Autodesk Inventor part; units mm, degrees
ref_plane "YZ Plane" through (0, 0, 0) normal (1, 0, 0) x (0, 1, 0)
ref_plane "XZ Plane" through (0, 0, 0) normal (0, 1, 0) x (-1, 0, 0)
ref_plane "XY Plane" through (0, 0, 0) normal (0, 0, 1) x (1, 0, 0)
sketch "Sketch1" plane through (0, 0, 0) normal (0, 1, 0) x (-1, 0, 0)
  line L0 (0, 0) -> (0, 15.8369)
  line L1 (0, 0) -> (20.1574, 0)
  line L2 (20.1574, 0) -> (20.1574, 7.7978)
  line L3 (20.1574, 7.7978) -> (0, 15.8369)
  dimension "d0" = 15.8369
  dimension "d1" = 20.1574
  dimension "d2" = 7.7978
extrude "Extrusion1" add sketch "Sketch1" along normal blind 3.236
sketch "Sketch2" plane through (0, 3.236, 0) normal (0, 1, 0) x (1, 0, 0)
  line L0 (-20.1574, -7.7978) -> (0, -15.8369)
  line L1 (-20.1574, 0) -> (-20.1574, -7.7978)
  line L2 (0, 0) -> (-20.1574, 0)
  line L3 (-20.1574, 0) -> (-20.1574, -7.7978)
  circle A0 centre (-16.2585, -3.8989) radius 2.4498
  dimension "d7" = 4.8997
extrude "Extrusion2" add sketch "Sketch2" along normal blind 1.9837
pattern_linear "Rectangular Pattern1" count 3 spacing 6.223 along (1, 0, 0) of "Extrusion2"
properties part number "other diagonal piece"
Verification items for the finished model (mm, model axes). A direction names the side the tool comes from. Coordinates: 2 decimals unless noted, no trailing zeros. Loops run counter-clockwise (first coordinate to the right, second up) from the corner with the lowest first, then second, coordinate; pieces in that order, holes last. Notation, with made-up numbers: (-33, 42.5) -> (-4, 42.5) arc R28 ccw to (-4, 70.5) -> close; hole circle Ø2 at (-32, -27.75). An arc over 180 degrees is marked (long way). Answer in a Markdown table with one row per item.
1) Scan lines: line 1 along X through (y, z) = (4.65, 4); line 2 along Y through (x, z) = (-7.5, 11); line 3 along Z through (x, y) = (-10.75, 4.85). Record each from-to range of solid material in increasing order. Write a range as from..to.
The answers:
| item | result |
|---|---|
| line 1 | x = -18.71..-13.81, -12.48..-7.59, -6.26..-1.36 |
| line 2 | y = 0..3.24 |
| line 3 | z = 1.56..6.24 |
2) Section check B-B (y = 3.85). Record the cut outline in (x, z).
The answers:
| item | result |
|---|---|
| outline | circle Ø4.9 at (-16.26, 3.9); circle Ø4.9 at (-10.04, 3.9); circle Ø4.9 at (-3.81, 3.9) |
3) Section check A-A (x = -2.75). Record the cut outline in (y, z).
The answers:
| item | result |
|---|---|
| outline | (0, 0) -> (3.24, 0) -> (3.24, 1.69) -> (5.22, 1.69) -> (5.22, 6.11) -> (3.24, 6.11) -> (3.24, 14.74) -> (0, 14.74) -> close |
4) Draft check along X on faces 1 (the face through (-10, 2, 0)), 2 (the face through (-4.13, 4.21, 6.33)), 3 (the face through (0, 2, 8)), 4 (the face through (-20.157, 2, 4)). Enter one of: released by +X, released by -X, zero draft, split by the parting line, or undercut.
The answers:
| item | result |
|---|---|
| face 1 | zero draft |
| face 2 | undercut |
| face 3 | released by +X |
| face 4 | released by -X |
5) Access from +Z, -Z, +X, -X, +Y, -Y to the whole of each face (thin tool, end or side, straight path). Record for faces 5 (the face through (-18.064, 4.214, 5.555)), 6 (the face through (-4, 5.22, 4)).
The answers:
| item | result |
|---|---|
| face 5 | +Y |
| face 6 | +Z, -Z, +X, -X, +Y |
6) Section check D-D (y = 1.35). Record the cut outline in (x, z).
The answers:
| item | result |
|---|---|
| outline | (-20.16, 0) -> (0, 0) -> (0, 15.84) -> (-20.16, 7.8) -> close |
7) Section check C-C (z = 7.5). Record the cut outline in (x, y).
The answers:
| item | result |
|---|---|
| outline | (-20.16, 0) -> (0, 0) -> (0, 3.24) -> (-20.16, 3.24) -> close |
